Source: CAD feature listing. Evaluate the final solid. Frame: model axes, mm. A direction names the side the tool comes from. Round coordinates to 2 decimals unless told otherwise and drop trailing zeros. Order: outer loops, then holes, each group sorted by start corner. A loop starts at its lowest first (then second) coordinate and runs counter-clockwise, first axis right, second up. Notation, with made-up numbers: M -6.5,1.5 L 51.5,1.5 A17 ccw 51.5,31.5 Z; hole C 75,25 d8. An arc over 180 degrees is marked long. Answer as CSV lines item,"result". Start each with the question number.
Item 1: Section query A-A on z = 0. Return the cut outline in (x, y).
Item 2: Section query B-B on x = 0. Return the cut outline in (y, z).
Item 3: Set-up query: faces 1 (the face through (9.5, 5, 0)), 2 (the face through (-11.56, 1.23, -15.08)). Return all of +Z, -Z, +X, -X, +Y, -Y with unobstructed straight access to the full face (end or side cutting, diameter ignored); none if empty.
Item 4: First-contact query: P1, Ø5.5, axis at y = 4.5, z = 3.5, coming from the +X side; P2, Ø1.5, axis at y = 4, z = 2, coming from the -X side; P3, Ø1.5, axis at x = -1.5, y = 6, coming from the +Z side; P4, Ø3, axis at y = 6.5, z = 3.5, coming from the +X side. Flat tips, straight axial feed; report the tip coordinate or a pass-through.
Item 5: Section query D-D on z = 9. Return the cut outline in (x, y).
Item 6: Pull-direction query (X, two-part tool) for faces 3 (the face through (0, 0, 8)), 4 (the face through (-4, 7.5, -6)), 5 (the face through (-5.17, 9.75, 12.47)); classes: +X half, -X half, draft (parallel to the pull), parting line (faces both ways), or undercut.
Item 7: Line query: line 1 (Y direction, x = -6, z = 6); line 2 (X direction, y = 10, z = 0); line 3 (X direction, y = 0.75, z = 0). Output: solid intervals per line, ascending. Write a range as [from, to].
Item 8: Section query C-C on y = 4. Return the cut outline in (x, z), plus the area to 3 significant figures.
from build123d import *

# Parameters (mm, degrees)
SKETCH1_R           = 19
BOSS_EXTRUDE1_DEPTH = 2.5
SKETCH2_R           = 13.5
BOSS_EXTRUDE2_DEPTH = 12
SKETCH3_R           = 7
CUT_EXTRUDE1_DEPTH  = 31.532769282
SKETCH4_W           = 19
SKETCH4_H           = 5
CUT_EXTRUDE2_DEPTH  = 17.5


with BuildPart() as part:
    # Sketch1 → Boss-Extrude1 (new body)
    with BuildSketch(Plane(origin=(0, 0, 0), x_dir=(1, 0, 0), z_dir=(0, 1, 0))):
        with Locations(Location((0, 0, 0), (0, 0, 270))):
            Circle(SKETCH1_R)
    extrude(amount=BOSS_EXTRUDE1_DEPTH)

    # Sketch2 → Boss-Extrude2 (add)
    with BuildSketch(Plane(origin=(0, 2.5, 0), x_dir=(1, 0, 0), z_dir=(0, 1, 0))):
        with Locations(Location((0, 0, 0), (0, 0, 270))):
            Circle(SKETCH2_R)
    extrude(amount=BOSS_EXTRUDE2_DEPTH)

    # Sketch3 → Cut-Extrude1 (cut, through all)
    with BuildSketch(Plane(origin=(0, 14.5, 0), x_dir=(1, 0, 0), z_dir=(0, 1, 0))):
        with Locations(Location((0, 0, 0), (0, 0, 270))):
            Circle(SKETCH3_R)
    extrude(amount=-CUT_EXTRUDE1_DEPTH, mode=Mode.SUBTRACT)

    # Sketch4 → Cut-Extrude2 (cut, symmetric)
    with BuildSketch(Plane.XY):
        with Locations((0, 5)):
            Rectangle(SKETCH4_W, SKETCH4_H)
    extrude(amount=CUT_EXTRUDE2_DEPTH, both=True, mode=Mode.SUBTRACT)


solid = part.part
Results:
1,outline,"M -19,0 L -7,0 L -7,2.5 L -9.5,2.5 L -9.5,7.5 L -7,7.5 L -7,14.5 L -13.5,14.5 L -13.5,2.5 L -19,2.5 Z; M 7,0 L 19,0 L 19,2.5 L 13.5,2.5 L 13.5,14.5 L 7,14.5 L 7,7.5 L 9.5,7.5 L 9.5,2.5 L 7,2.5 Z"
2,outline,"M 0,-19 L 2.5,-19 L 2.5,-7 L 0,-7 Z; M 0,7 L 2.5,7 L 2.5,19 L 0,19 Z; M 7.5,-13.5 L 14.5,-13.5 L 14.5,-7 L 7.5,-7 Z; M 7.5,7 L 14.5,7 L 14.5,13.5 L 7.5,13.5 Z"
3,face 1,"+Z, -Z"
3,face 2,"+Y, -Y"
4,P1,"x = 18.93"
4,P2,"x = -13.44"
4,P3,"through"
4,P4,"x = 13.35"
5,outline,"M -16.73,0 L 16.73,0 L 16.73,2.5 L 10.06,2.5 L 10.06,14.5 L -10.06,14.5 L -10.06,2.5 L -16.73,2.5 Z; hole M -9.5,2.5 L 9.5,2.5 L 9.5,7.5 L -9.5,7.5 Z"
6,face 3,"draft"
6,face 4,"undercut"
6,face 5,"parting line"
7,line 1,"[0, 2.5], [7.5, 14.5]"
7,line 2,"[-13.5, -7], [7, 13.5]"
7,line 3,"[-19, -7], [7, 19]"
8,outline,"M -9.5,-9.59 L -9.5,9.59 A13.5 ccw Z; M 9.5,-9.59 A13.5 ccw 9.5,9.59 Z"
8,area,"106 mm^2"
